Input: dimensioned drawing with shaded views. Units: mm. Origin: part minimum x, y, z. A direction names the side the tool comes from. Give positions to 0.01 mm unless a question says otherwise; leave off trailing zeros. Write each loop counter-clockwise with the first axis right and the second up, starting at its lowest first coordinate (ties: lowest second). Pieces come first, ordered by that corner, then holes.
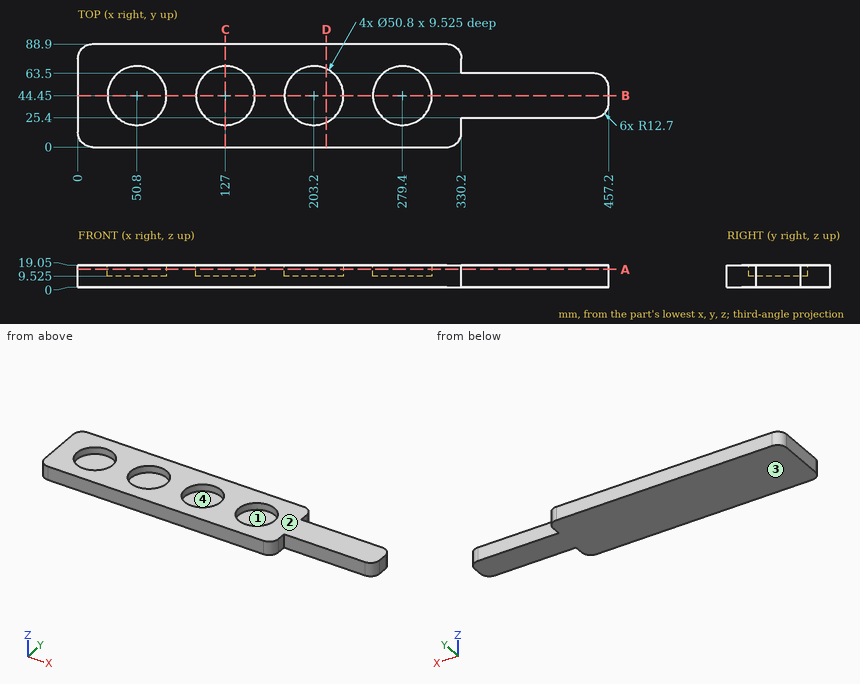
1. Access query for the marked faces 3 and 4. Directions: +Z, -Z, +X, -X, +Y, -Y. A direction counts if a zero-diameter tool reaches every point of the face in a straight line with its end or side. Return the directions, or none.
2. Cut plane D-D, the plane x = 214. Return the cut outline in (y, z) (3 decimals).
3. Mould query, pull axis X, two halves, no side actions, for the marked faces 1 and 2. Classes: +X half, -X half, draft (parallel to the pull), parting line (faces both ways), or undercut.
4. Cut plane B-B, the plane y = 44.45. Return the cut outline in (x, z) (3 decimals).
5. Cut plane C-C, the plane x = 127. Return the cut outline in (y, z) (3 decimals), then the cut area to 3 significant figures.
6. Line query: L1, parallel to Y at x = 50.8, z = 14; L2, parallel to Y at x = 331, z = 12; L3, parallel to X at y = 64, z = 14.25. Output: solid intervals per line, ascending.
7. Cut plane A-A, the plane z = 15.5. Return the cut outline in (x, y).
8. Contact query for flat-ended pins moving along their axis: P1, Ø9.5, axis at x = 387, z = 11, coming from the -Y side; P2, Ø15, axis at x = 285.5, y = 45, coming from the +Z side (3 decimals); P3, Ø6.5, axis at y = 21.5, z = 5, coming from the +X side. Output: stop coordinate, or through.
Response values:
1. face 3: -Z, +X, -X, +Y, -Y
1. face 4: +Z
2. outline: (0, 0) - (88.9, 0) - (88.9, 19.05) - (67.44, 19.05) - (67.44, 9.525) - (21.46, 9.525) - (21.46, 19.05) - (0, 19.05) - close
3. face 1: undercut
3. face 2: draft
4. outline: (0, 0) - (457.2, 0) - (457.2, 19.05) - (304.8, 19.05) - (304.8, 9.525) - (254, 9.525) - (254, 19.05) - (228.6, 19.05) - (228.6, 9.525) - (177.8, 9.525) - (177.8, 19.05) - (152.4, 19.05) - (152.4, 9.525) - (101.6, 9.525) - (101.6, 19.05) - (76.2, 19.05) - (76.2, 9.525) - (25.4, 9.525) - (25.4, 19.05) - (0, 19.05) - close
5. outline: (0, 0) - (88.9, 0) - (88.9, 19.05) - (69.85, 19.05) - (69.85, 9.525) - (19.05, 9.525) - (19.05, 19.05) - (0, 19.05) - close
5. area: 1,210 mm2
6. L1: y = 0 to 19.05, 69.85 to 88.9
6. L2: y = 25.4 to 63.5
6. L3: x = 0 to 34.58, 67.02 to 110.78, 143.22 to 186.98, 219.42 to 263.18, 295.62 to 330.2
7. outline: (0, 12.7) arc R12.7 ccw to (12.7, 0) - (317.5, 0) arc R12.7 ccw to (330.2, 12.7) - (330.2, 25.4) - (444.5, 25.4) arc R12.7 ccw to (457.2, 38.1) - (457.2, 50.8) arc R12.7 ccw to (444.5, 63.5) - (330.2, 63.5) - (330.2, 76.2) arc R12.7 ccw to (317.5, 88.9) - (12.7, 88.9) arc R12.7 ccw to (0, 76.2) - close; hole circle Ø50.8 at (50.8, 44.45); hole circle Ø50.8 at (127, 44.45); hole circle Ø50.8 at (203.2, 44.45); hole circle Ø50.8 at (279.4, 44.45)
8. P1: stops at y = 25.4
8. P2: stops at z = 9.525
8. P3: stops at x = 330.2
